Autodesk Inventor part; units mm, degrees
ref_plane "YZ Plane" through (0, 0, 0) normal (1, 0, 0) x (0, 1, 0)
ref_plane "XZ Plane" through (0, 0, 0) normal (0, 1, 0) x (-1, 0, 0)
ref_plane "XY Plane" through (0, 0, 0) normal (0, 0, 1) x (1, 0, 0)
sketch "スケッチ1" plane through (0, 0, 0) normal (0, 0, 1) x (1, 0, 0)
  circle A0 centre (0, 0) radius 65 construction
  line L0 (-42.5, 65) -> (42.5, 65) construction
  line L1 (42.5, 65) -> (42.5, -65) construction
  line L2 (42.5, -65) -> (-42.5, -65) construction
  line L3 (-42.5, -65) -> (-42.5, 65) construction
  arc A1 (42.5, 49.1808) -> (-42.5, 49.1808) centre (0, 0) ccw
  line L4 (-42.5, 49.1808) -> (-42.5, -49.1808)
  line L5 (42.5, 49.1808) -> (42.5, -49.1808)
  arc A2 (-42.5, -49.1808) -> (42.5, -49.1808) centre (0, 0) ccw
  point P0 (0, 65)
  dimension "d0" = 130
  dimension "d1" = 85
extrude "基板" add sketch "スケッチ1" along normal blind 1.6
sketch "スケッチ4" plane through (0, 0, 1.6) normal (0, 0, 1) x (1, 0, 0)
  line L0 (0, -55.1622) -> (0, 55.1622) construction
  line L1 (42.5, -49.1808) -> (42.5, 49.1808) construction
  circle A0 centre (0, 0) radius 60 construction
  line L2 (0, 0) -> (36.3616, 43.334) construction
  line L3 (0, 0) -> (56.5685, 0) construction
  point P0 (38.5, -46.019)
  point P1 (-38.5, -46.019)
  point P2 (38.5673, 45.9627)
  point P3 (-38.5673, 45.9627)
  dimension "d27" = 4
  dimension "d29" = 120
  dimension "d30" = 50
hole "スペーサ取付穴" at (38.5, -46.019, 1.6) at (-38.5, -46.019, 1.6) at (38.5673, 45.9627, 1.6) at (-38.5673, 45.9627, 1.6) direction (0, 0, -1) diameter 3.2 end through all
sketch "スケッチ6" plane through (0, 0, 1.6) normal (0, 0, 1) x (1, 0, 0)
  line L0 (-42.5, 49.1808) -> (-42.5, -49.1808)
  line L1 (-42.5, 9.5) -> (-25, 9.5)
  line L2 (-25, 9.5) -> (-25, -9.5)
  line L3 (-25, -9.5) -> (-42.5, -9.5)
  line L4 (-42.5, -9.5) -> (-42.5, 9.5)
  line L5 (42.5, 9.5) -> (25, 9.5)
  line L6 (25, 9.5) -> (25, -9.5)
  line L7 (25, -9.5) -> (42.5, -9.5)
  line L8 (42.5, -9.5) -> (42.5, 9.5)
  line L9 (42.5, -49.1808) -> (42.5, 49.1808)
  point P0 (0, 0)
  point P1 (-25, 0)
  dimension "d43" = 19
  dimension "d44" = 17.5
extrude "モータ用切欠き" cut sketch "スケッチ6" against normal through all
fillet "フィレット1" radius 1.5 4 edges at (-25, 9.5, 0.8) (-25, -9.5, 0.8) (25, 9.5, 0.8) (25, -9.5, 0.8)
properties part number "BaseBoard3"
Build history of the part. All positions in model axes, mm. Give positions to 0.01 mm unless a question says otherwise; leave off trailing zeros. Loops run counter-clockwise (first coordinate to the right, second up) from the corner with the lowest first, then second, coordinate; pieces in that order, holes last.
1) Band-saw the part on A-A on y = 46. List the corners of the cut face in (x, z).
Values follow:
outline: (-42.5, 0) - (-40.17, 0) - (-40.17, 1.6) - (-42.5, 1.6) - close; (-36.97, 0) - (36.97, 0) - (36.97, 1.6) - (-36.97, 1.6) - close; (40.17, 0) - (42.5, 0) - (42.5, 1.6) - (40.17, 1.6) - close
2) Band-saw the part on D-D on x = 15. List the corners of the cut face in (y, z), then the cut area to 3 significant figures.
Values follow:
outline: (-63.25, 0) - (63.25, 0) - (63.25, 1.6) - (-63.25, 1.6) - close
area: 202 mm2
3) Drop a flat-ended pin along its axis: P1, Ø0.8, axis at x = 33, z = 0.5, coming from the -Y side. Give the stop position or say it passes through.
Values follow:
P1: stops at y = -56.23
4) Probe line 1 along Y through (x, z) = (-37.5, 0.3); line 2 along Y through (x, z) = (-33, 1); line 3 along Y through (x, z) = (1.5, 0.35). List the from-to ranges inside material, lowest first.
Values follow:
line 1: y = -53.09 to -47.27, -44.77 to -9.5, 9.5 to 44.77, 47.15 to 53.09
line 2: y = -56 to -9.5, 9.5 to 56
line 3: y = -64.98 to 64.98
5) Two-plate mould, pull along Y, no slides. Class faces 1 (the face through (38.087, 44.437, 0.789)), 2 (the face through (-0.649, 64.997, 0.789)), 3 (the face through (-1, 1, 0)): released by +Y, released by -Y, zero draft, split by the parting line, or undercut.
Values follow:
face 1: undercut
face 2: released by +Y
face 3: zero draft
6) Band-saw the part on C-C on z = 0.8. List the corners of the cut face in (x, y), then the cut area to 3 significant figures.
Values follow:
outline: (-42.5, -49.18) arc R65 ccw to (42.5, -49.18) - (42.5, -9.5) - (26.5, -9.5) arc R1.5 cw to (25, -8) - (25, 8) arc R1.5 cw to (26.5, 9.5) - (42.5, 9.5) - (42.5, 49.18) arc R65 ccw to (-42.5, 49.18) - (-42.5, 9.5) - (-26.5, 9.5) arc R1.5 cw to (-25, 8) - (-25, -8) arc R1.5 cw to (-26.5, -9.5) - (-42.5, -9.5) - close; hole circle Ø3.2 at (-38.57, 45.96); hole circle Ø3.2 at (-38.5, -46.02); hole circle Ø3.2 at (38.5, -46.02); hole circle Ø3.2 at (38.57, 45.96)
area: 9,510 mm2
7) Band-saw the part on B-B on x = 29. List the corners of the cut face in (y, z).
Values follow:
outline: (-58.17, 0) - (-9.5, 0) - (-9.5, 1.6) - (-58.17, 1.6) - close; (9.5, 0) - (58.17, 0) - (58.17, 1.6) - (9.5, 1.6) - close
